Can you work these out from the model? Positions are in its coordinate system, mm. Coordinates: 2 decimals unless noted, no trailing zeros. Order: outer loops, then holes, each group sorted by start corner. A loop starts at its lowest first (then second) coordinate and runs counter-clockwise, first axis right, second up. Notation, with made-up numbers: (75, -20) -> (134, -20) arc R23 cw to (134, -5) -> close; hole circle Ø9 at (79.25, 64.5). An arc over 180 degrees is marked (long way). Answer in a Markdown table with one row per item.
```python
from build123d import *

# Parameters (mm, degrees)
SKETCH1_W           = 114.261019043
SKETCH1_H           = 76.109285411
BOSS_EXTRUDE1_DEPTH = 12.7
SKETCH2_R           = 6.465438967
CUT_EXTRUDE1_DEPTH  = 28.194
SKETCH3_R           = 6.272780884
CUT_EXTRUDE2_DEPTH  = 31.242


with BuildPart() as part:
    # Sketch1 → Boss-Extrude1 (new body)
    with BuildSketch(Plane(origin=(0, 0, 0), x_dir=(1, 0, 0), z_dir=(0, 1, 0))):
        with Locations((-57.130509522, 38.054642706)):
            Rectangle(SKETCH1_W, SKETCH1_H)
    extrude(amount=-BOSS_EXTRUDE1_DEPTH)

    # Sketch2 → Cut-Extrude1 (cut)
    with BuildSketch(Plane.XZ.offset(12.7)):
        with Locations(Location((-10.03566432, -14.029659272, 0), (0, 0, 270))):
            Circle(SKETCH2_R)
    extrude(amount=-CUT_EXTRUDE1_DEPTH, mode=Mode.SUBTRACT)

    # Sketch3 → Cut-Extrude2 (cut)
    with BuildSketch(Plane.XZ.offset(12.7)):
        with Locations(Location((-9.80844034, -62.176336471, 0), (0, 0, 270))):
            Circle(SKETCH3_R)
    extrude(amount=-CUT_EXTRUDE2_DEPTH, mode=Mode.SUBTRACT)


solid = part.part
```
(1) Suppose I cut it at A-A (z = -65). Please give me the cut outline in (x, y), and give its area (3 significant figures).
Response values:
| item | result |
|---|---|
| outline | (-114.26, -12.7) -> (-15.41, -12.7) -> (-15.41, 0) -> (-114.26, 0) -> close; (-4.21, -12.7) -> (0, -12.7) -> (0, 0) -> (-4.21, 0) -> close |
| area | 1,310 mm2 |
(2) I need wall thicknesses on line 1 (X direction, y = -2.25, z = -62); line 2 (Z direction, x = -14, y = -6.5); line 3 (X direction, y = -11.5, z = -10). Which ranges of each line are inside material? Lowest first, please. Write a range as [from, to].
Response values:
| item | result |
|---|---|
| line 1 | [-114.26, -16.08], [-3.54, 0] |
| line 2 | [-76.11, -66.84], [-57.51, -19.14], [-8.92, 0] |
| line 3 | [-114.26, -15.09], [-4.98, 0] |
(3) Suppose I cut it at B-B (y = -4.5). Please give me the cut outline in (x, z).
Response values:
| item | result |
|---|---|
| outline | (-114.26, -76.11) -> (0, -76.11) -> (0, 0) -> (-114.26, 0) -> close; hole circle Ø12.93 at (-10.04, -14.03); hole circle Ø12.55 at (-9.81, -62.18) |
(4) Suppose I cut it at C-C (z = -12). Please give me the cut outline in (x, y), and give its area (3 significant figures).
Response values:
| item | result |
|---|---|
| outline | (-114.26, -12.7) -> (-16.17, -12.7) -> (-16.17, 0) -> (-114.26, 0) -> close; (-3.9, -12.7) -> (0, -12.7) -> (0, 0) -> (-3.9, 0) -> close |
| area | 1,300 mm2 |
(5) We'd pull the mould along X, two halves only. Please class faces 1 (the cylindrical face through (-8.1, -6.4, -20.2)), 2 (the flat face through (-114.261, -6, -38)), 3 (the flat face through (-58, -6, -76.109)), 4 (the flat face through (0, -6, -38)): +X half, -X half, draft (parallel to the pull), parting line (faces both ways), or undercut.
Response values:
| item | result |
|---|---|
| face 1 | undercut |
| face 2 | -X half |
| face 3 | draft |
| face 4 | +X half |
